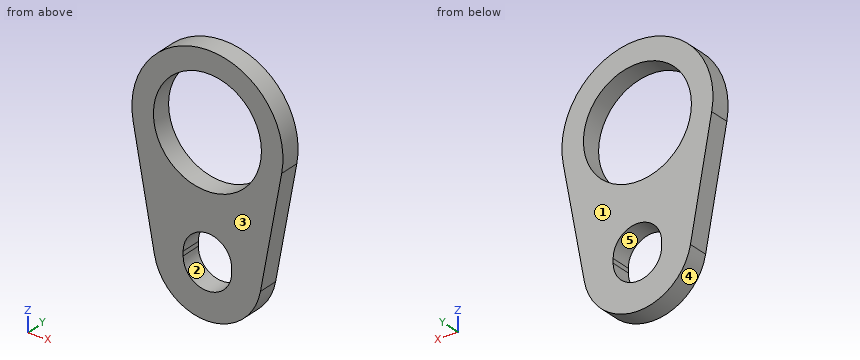
from build123d import *

# Parameters (mm, degrees)
F0_R     = 50.0507
F1_DEPTH = 19.05


with BuildPart() as f1:
    # F0 (on Front) → F1 (new body)
    with BuildSketch(Plane.XZ):
        with BuildLine():
            Line((49.1666083018, -119.0909090909), (68.8332516225, -12.7272727273))
            ThreePointArc((68.8332516225, -12.7272727273), (0, 70), (-68.8332516225, -12.7272727273))
            Line((-68.8332516225, -12.7272727273), (-49.1666083018, -119.0909090909))
            ThreePointArc((-49.1666083018, -119.0909090909), (0, -160), (49.1666083018, -119.0909090909))
        make_face()
        with BuildLine():
            Line((-22.5, -112), (-22.5, -108))
            ThreePointArc((-22.5, -108), (0, -85.5), (22.5, -108))
            Line((22.5, -108), (22.5, -112))
            ThreePointArc((22.5, -112), (0, -134.5), (-22.5, -112))
        make_face(mode=Mode.SUBTRACT)
        Circle(F0_R, mode=Mode.SUBTRACT)
    extrude(amount=F1_DEPTH)


solid = f1.part
Here's how the part is built. I have some questions about the finished solid (model axes, mm). Face numbers are marked on the shaded views. A direction names the side the tool comes from. Round coordinates to 2 decimals unless told otherwise and drop trailing zeros. Write each loop counter-clockwise with the first axis right and the second up, starting at its lowest first coordinate (ties: lowest second). Pieces come first, ordered by that corner, then holes.
1. Suppose I cut it at B-B (x = 0). List the corners of the cut face in (y, z) for me.
2. Suppose I cut it at C-C (y = -11.75). List the corners of the cut face in (x, z) for me, and give its area (3 significant figures).
3. For the marked faces 1 and 2, which set-ups out of +Z, -Z, +X, -X, +Y, -Y let a thin tool reach every point of the face, with its end or its side?
4. Suppose I cut it at A-A (z = 0). List the corners of the cut face in (x, y) for me, and give its area (3 significant figures).
5. I need wall thicknesses on L1, parallel to Z at x = 0, y = -6.25; L2, parallel to Z at x = -10, y = -11; L3, parallel to Z at x = -29, y = -16.75. Which ranges of each line are inside material? Lowest first, please.
6. Will these pins go through, and if not, where does the flat tip stop? pin 1 Ø4 at (x, y) = (15, -3) entering from +Z; pin 2 Ø2 at (y, z) = (-9, -109.5) entering from -X; pin 3 Ø10 at (x, y) = (-16.5, -7) entering from +Z.
7. If we mould it in two halves opening along X, with no side actions, what happens to the marked faces 3, 4 and 5? For each: released by +X, released by -X, zero draft, split by the parting line, or undercut.
8. Suppose I cut it at D-D (x = -45.5). List the corners of the cut face in (y, z) for me, and give its area (3 significant figures).
Answer sheet:
1. outline: (-19.05, -160) - (0, -160) - (0, -134.5) - (-19.05, -134.5) - close; (-19.05, -85.5) - (0, -85.5) - (0, -50.05) - (-19.05, -50.05) - close; (-19.05, 50.05) - (0, 50.05) - (0, 70) - (-19.05, 70) - close
2. outline: (-68.83, -12.73) - (-49.17, -119.09) arc R50 ccw to (49.17, -119.09) - (68.83, -12.73) arc R70 ccw (long way) to start; hole circle Ø100.1 at (0, 0); hole (-22.5, -112) arc R22.5 ccw to (22.5, -112) - (22.5, -108) arc R22.5 ccw to (-22.5, -108) - close
2. area: 15,400 mm2
3. face 1: +Z, -Z, +X, -X, +Y
3. face 2: +Y, -Y
4. outline: (-70, -19.05) - (-50.05, -19.05) - (-50.05, 0) - (-70, 0) - close; (50.05, -19.05) - (70, -19.05) - (70, 0) - (50.05, 0) - close
4. area: 760 mm2
5. L1: z = -160 to -134.5, -85.5 to -50.05, 50.05 to 70
5. L2: z = -158.99 to -132.16, -87.84 to -49.04, 49.04 to 69.28
5. L3: z = -150.73 to -40.79, 40.79 to 63.71
6. pin 1: stops at z = 68.78
6. pin 2: stops at x = -51.12
6. pin 3: stops at z = 69.05
7. face 3: zero draft
7. face 4: split by the parting line
7. face 5: undercut
8. outline: (-19.05, -130.73) - (0, -130.73) - (0, -20.85) - (-19.05, -20.85) - close; (-19.05, 20.85) - (0, 20.85) - (0, 53.2) - (-19.05, 53.2) - close
8. area: 2,710 mm2
